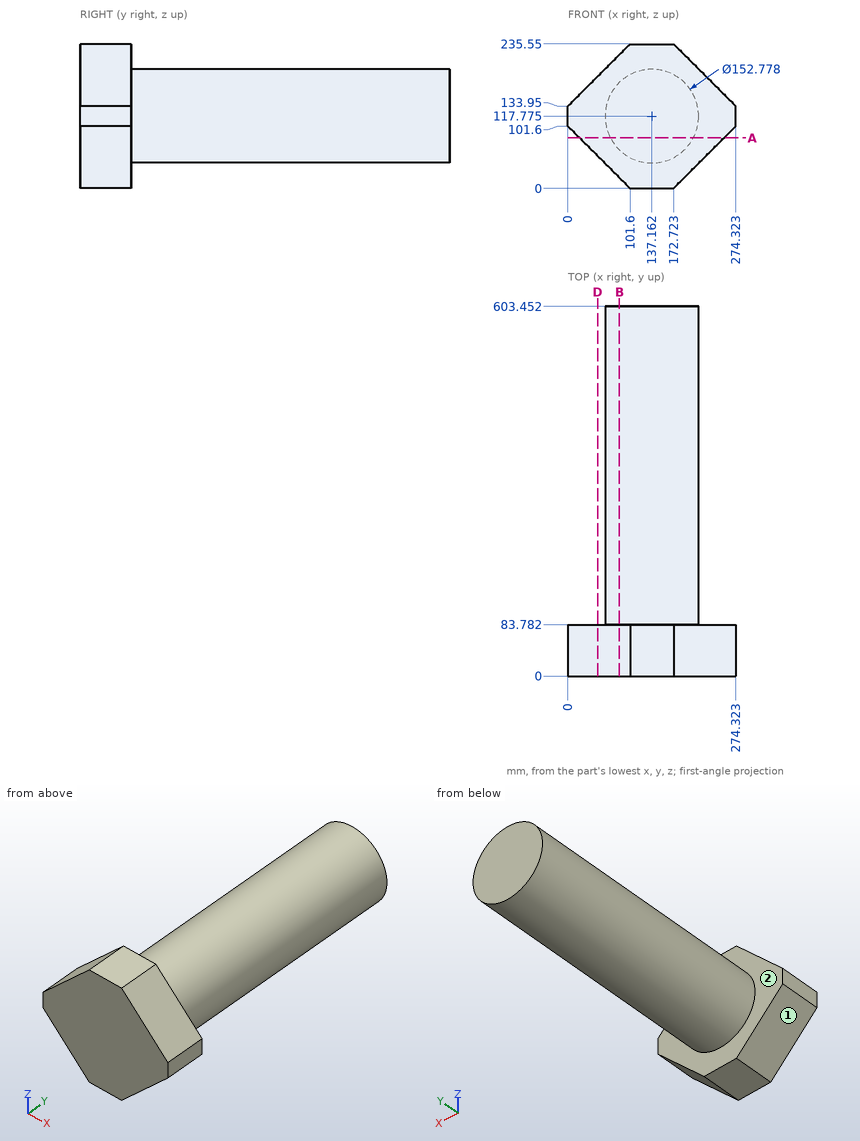
Geometry check sheet. Reference: drawing and pictorial views, mm from the part's lowest x, y, z. A direction names the side the tool comes from. Give positions to 0.01 mm unless a question says otherwise; leave off trailing zeros. Write each loop counter-clockwise with the first axis right and the second up, starting at its lowest first coordinate (ties: lowest second). Pieces come first, ordered by that corner, then holes. Notation, with made-up numbers: (80.5, 43) - (120.5, 43) arc R26 cw to (120.5, 58) - close; hole circle Ø10 at (39.5, 35.5). An arc over 180 degrees is marked (long way). Put each result on its own line as item: value.
Q1. Section check B-B on x = 84. Record the cut outline in (y, z), and give its area (3 significant figures).
Result:
outline: (0, 17.6) - (83.78, 17.6) - (83.78, 62.92) - (603.45, 62.92) - (603.45, 172.63) - (83.78, 172.63) - (83.78, 217.95) - (0, 217.95) - close
area: 73,800 mm2
Q2. Scan lines: probe 1 along Y at (x, z) = (12.5, 135); probe 2 along Z at (x, y) = (111.5, 540) (1 decimal); probe 3 along X at (y, z) = (379.5, 149) (1 decimal). Record each from-to range of solid material in increasing order. Write a range as from..to.
Result:
probe 1: 0..83.78
probe 2: 45.8..189.7
probe 3: 67.4..206.9
Q3. Depth check by flat-ended pin: P1, Ø1, axis at x = 177, y = 310, coming from the +Z side (1 decimal); P2, Ø2, axis at x = 142, y = 257.5, coming from the +Z side; P3, Ø10, axis at y = 444, z = 138.5, coming from the -X side. Enter the tip coordinate at first touch or a pass-through.
Result:
P1: z = 183.3
P2: z = 194.07
P3: x = 62.41
Q4. Set-up check for the marked faces 1 and 2: record each of +Z, -Z, +X, -X, +Y, -Y from which the full face is reachable in a straight line by a thin tool's end or side.
Result:
face 1: -Z, -X, +Y, -Y
face 2: +Y
Q5. Section check A-A on z = 82.5. Record the cut outline in (x, y) (1 decimal).
Result:
outline: (19.1, 0) - (255.2, 0) - (255.2, 83.8) - (204.9, 83.8) - (204.9, 603.5) - (69.4, 603.5) - (69.4, 83.8) - (19.1, 83.8) - close
Q6. Section check D-D on x = 48.5. Record the cut outline in (y, z).
Result:
outline: (0, 53.1) - (83.78, 53.1) - (83.78, 182.45) - (0, 182.45) - close
